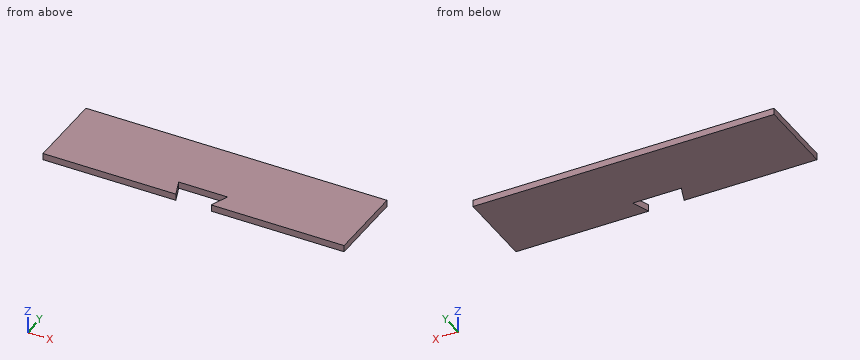
from build123d import *

# Parameters (mm, degrees)
F0_W     = 863.6
F0_H     = 228.6
F1_DEPTH = 19.05
F3_DEPTH = 19.051


with BuildPart() as f1:
    # F0 (on Top) → F1 (new body)
    with BuildSketch(Plane.XY):
        with Locations((0, -114.3)):
            Rectangle(F0_W, F0_H)
    extrude(amount=F1_DEPTH)

    # F2 (on face) → F3 (cut, through all)
    with BuildSketch(Plane.XY.offset(19.05)):
        Polygon((-69.85, -177.8), (-50.8, -228.6), (50.8, -228.6), (69.85, -177.8), align=None)
    extrude(amount=-F3_DEPTH, mode=Mode.SUBTRACT)


solid = f1.part
Could you check a few things on this model? Use its own coordinates, in mm. Coordinates: 2 decimals unless noted, no trailing zeros. Order: outer loops, then holes, each group sorted by start corner. A loop starts at its lowest first (then second) coordinate and runs counter-clockwise, first axis right, second up. Notation, with made-up numbers: (84.25, 64.25) -> (94.25, 64.25) arc R22 ccw to (94.25, 70.25) -> close; hole circle Ø9 at (65.25, 39). An arc over 180 degrees is marked (long way). One line per item, written item: value. Start each with the question number.
1) Imagine slicing it at B-B on x = 61. List the corners of the cut face in (y, z) for me, plus the area to 3 significant figures.
2) If I drill on L1, parallel to Y at x = -12, z = 8; L2, parallel to X at y = -190.5, z = 16.25; L3, parallel to X at y = -218.5, z = 11.5, over which ranges is the centre line in solid material (lowest first)? Write a range as [from, to].
3) Imagine slicing it at D-D on x = -40. List the corners of the cut face in (y, z) for me, plus the area to 3 significant figures.
4) Imagine slicing it at A-A on y = -209. List the corners of the cut face in (x, z) for me.
5) Imagine slicing it at C-C on z = 12.25. List the corners of the cut face in (x, y) for me, plus the area to 3 significant figures.
6) I'm going to push a flat-ended pin straight in: pin 1 (1 mm diameter, centred on x = -20, z = 7, fed in from -Y). Where does the tip first touch, or does it pass through?
Answer list:
1. outline: (-228.6, 0) -> (-201.4, 0) -> (-201.4, 19.05) -> (-228.6, 19.05) -> close; (-177.8, 0) -> (0, 0) -> (0, 19.05) -> (-177.8, 19.05) -> close
1. area: 3,910 mm2
2. L1: y = [-177.8, 0]
2. L2: x = [-431.8, -65.09], [65.09, 431.8]
2. L3: x = [-431.8, -54.59], [54.59, 431.8]
3. outline: (-177.8, 0) -> (0, 0) -> (0, 19.05) -> (-177.8, 19.05) -> close
3. area: 3,390 mm2
4. outline: (-431.8, 0) -> (-58.15, 0) -> (-58.15, 19.05) -> (-431.8, 19.05) -> close; (58.15, 0) -> (431.8, 0) -> (431.8, 19.05) -> (58.15, 19.05) -> close
5. outline: (-431.8, -228.6) -> (-50.8, -228.6) -> (-69.85, -177.8) -> (69.85, -177.8) -> (50.8, -228.6) -> (431.8, -228.6) -> (431.8, 0) -> (-431.8, 0) -> close
5. area: 191,000 mm2
6. pin 1: stops at y = -177.8
